Here's how the part is built. I have some questions about the finished solid (model axes, mm). Face numbers are marked on the shaded views. A direction names the side the tool comes from. Coordinates: 2 decimals unless noted, no trailing zeros. Write each loop counter-clockwise with the first axis right and the second up, starting at its lowest first coordinate (ties: lowest second). Pieces come first, ordered by that corner, then holes.
Autodesk Inventor part; units mm, degrees
ref_plane "YZ Plane" through (0, 0, 0) normal (1, 0, 0) x (0, 1, 0)
ref_plane "XZ Plane" through (0, 0, 0) normal (0, 1, 0) x (-1, 0, 0)
ref_plane "XY Plane" through (0, 0, 0) normal (0, 0, 1) x (1, 0, 0)
sketch "Sketch1" plane through (0, 0, 0) normal (0, 1, 0) x (-1, 0, 0)
  line L0 (110, -80) -> (-110, -80)
  line L1 (-110, -80) -> (-110, 80)
  line L2 (-110, 80) -> (110, 80)
  line L3 (110, 80) -> (110, -80)
  line L4 (320.2117, -53.5522) -> (168.036, -53.5522) construction
  line L5 (168.036, -53.5522) -> (168.036, 90.1689) construction
  line L6 (168.036, 90.1689) -> (320.2117, 90.1689) construction
  line L7 (320.2117, 90.1689) -> (320.2117, -53.5522) construction
  line L8 (124.3, -89.75) -> (-124.3, -89.75) construction
  line L9 (-124.3, -89.75) -> (-124.3, 89.75) construction
  line L10 (-124.3, 89.75) -> (124.3, 89.75) construction
  line L11 (124.3, 89.75) -> (124.3, -89.75) construction
  line L12 (124.3, -89.75) -> (-124.3, 89.75) construction
  line L13 (-124.3, -89.75) -> (124.3, 89.75) construction
  line L14 (-152.4, -107.95) -> (152.4, -107.95)
  line L15 (152.4, -107.95) -> (152.4, 107.95)
  line L16 (152.4, 107.95) -> (-152.4, 107.95)
  line L17 (-152.4, 107.95) -> (-152.4, -107.95)
  line L18 (-152.4, -107.95) -> (152.4, 107.95) construction
  line L19 (152.4, -107.95) -> (-152.4, 107.95) construction
  line L20 (177.8, 133.35) -> (177.8, -133.35)
  line L21 (177.8, -133.35) -> (-177.8, -133.35)
  line L22 (-177.8, -133.35) -> (-177.8, 133.35)
  line L23 (-177.8, 133.35) -> (177.8, 133.35)
  point P0 (0, 0)
  dimension "d11" = 220
  dimension "d12" = 160
  dimension "d15" = 248.6
  dimension "d16" = 179.5
  dimension "d18" = 304.8
  dimension "d19" = 215.9
  dimension "d22" = 25.4
extrude "Top" add sketch "Sketch1" along normal blind 25.4 contours L17 L16 L15 L14 | L20 L21 L22 L23
sketch "Sketch3" plane through (177.8, 0, 133.35) normal (1, 0, 0) x (0, 0, -1)
  line L0 (0, 0) -> (0, 25.4)
  line L1 (266.7, 0) -> (266.7, 25.4)
  line L2 (0, 0) -> (266.7, 0)
  line L3 (266.7, 0) -> (266.7, -266.7)
  line L4 (266.7, -266.7) -> (0, -266.7)
  line L5 (0, -266.7) -> (0, 0)
  point P0 (133.35, 0)
  dimension "d25" = 266.7
extrude "Right" add sketch "Sketch3" against normal blind 50.8
sketch "Sketch4" plane through (-177.8, 0, -133.35) normal (-1, 0, 0) x (0, 0, 1)
  line L0 (0, 0) -> (0, 25.4)
  line L1 (266.7, -266.7) -> (266.7, 0)
  line L2 (0, 0) -> (266.7, 0)
  line L3 (266.7, 0) -> (266.7, -266.7)
  line L4 (266.7, -266.7) -> (0, -266.7)
  line L5 (0, -266.7) -> (0, 0)
  point P0 (133.35, 0)
  dimension "d28" = 266.7
extrude "Left" add sketch "Sketch4" against normal blind 50.8
sketch "Sketch5" plane through (0, 0, 0) normal (1, 0, 0) x (0, 1, 0)
  line L0 (-266.7, -133.35) -> (25.4, -133.35)
  line L1 (-266.7, 133.35) -> (-266.7, -133.35)
  line L2 (0, -133.35) -> (-266.7, 133.35)
  line L3 (-266.7, 133.35) -> (-275.6803, 124.3697)
  line L4 (-275.6803, 124.3697) -> (-8.9803, -142.3303)
  line L5 (-8.9803, -142.3303) -> (0, -133.35)
  point P0 (0, 0)
  dimension "d31" = 12.7
extrude "Plexiglass Cut" cut sketch "Sketch5" along normal mid plane 304.8 contours L4 L1 L2 L0 | L0 L5 L4 | L4 L3 L1
sketch "Sketch6" plane through (-177.8, -266.7, -133.35) normal (0, -1, 0) x (1, 0, 0)
  line L0 (0, 0) -> (0, 266.7)
  line L1 (355.6, 0) -> (0, 0)
  line L2 (0, 266.7) -> (355.6, 266.7)
  line L3 (355.6, 266.7) -> (355.6, 0)
  line L4 (355.6, 0) -> (0, 0)
  line L5 (0, 0) -> (0, 266.7)
  point P0 (177.8, 133.35)
extrude "Bottom" add sketch "Sketch6" along normal blind 25.4
sketch "Sketch9" plane through (0, 25.4, 0) normal (0, 1, 0) x (1, 0, 0)
  line L0 (177.8, -133.35) -> (127, -133.35)
  line L1 (177.8, 133.35) -> (-177.8, 133.35)
  line L2 (177.8, -133.35) -> (-177.8, -133.35)
  line L3 (-177.8, -133.35) -> (-177.8, 133.35)
  line L4 (-177.8, 133.35) -> (177.8, 133.35)
  line L5 (177.8, 133.35) -> (177.8, -133.35)
  point P0 (0, 0)
extrude "Top Flattening" cut sketch "Sketch9" against normal blind 22.4
sketch "Sketch10" plane through (0, 3, 0) normal (0, 1, 0) x (1, 0, 0)
  line L0 (-177.8, -133.35) -> (-177.8, 133.35)
  line L1 (-155.4106, 133.35) -> (-177.8, 133.35)
  line L2 (-177.8, 133.35) -> (-177.8, -133.35)
  line L3 (-177.8, -133.35) -> (-155.4106, -133.35)
  line L4 (-155.4106, -133.35) -> (-155.4106, 133.35)
  line L5 (177.8, 133.35) -> (177.8, -133.35)
  line L6 (177.8, -133.35) -> (155.4106, -133.35)
  line L7 (155.4106, -133.35) -> (155.4106, 133.35)
  line L8 (155.4106, 133.35) -> (177.8, 133.35)
  line L9 (152.4, -115.3895) -> (152.4, 133.35)
  point P0 (0, 0)
  point P1 (-177.8, 0)
  dimension "d48" = 22.3894
  dimension "d49" = 22.3894
extrude "Outer Side Flattening" cut sketch "Sketch10" against normal through all
sketch "Sketch11" plane through (-177.8, -292.1, -133.35) normal (0, -1, 0) x (1, 0, 0)
  line L0 (22.3894, 0) -> (333.2106, 0)
  line L1 (333.2106, 0) -> (22.3894, 0)
  line L2 (22.3894, 0) -> (22.3894, 266.7)
  line L3 (22.3894, 266.7) -> (333.2106, 266.7)
  line L4 (333.2106, 266.7) -> (333.2106, 0)
  point P0 (177.8, 133.35)
extrude "Bottom Flattening" cut sketch "Sketch11" against normal blind 22.4
sketch "Sketch12" plane through (155.4106, 3, -133.35) normal (0, 0, -1) x (-1, 0, 0)
  line L0 (155.4106, -3) -> (155.4106, -269.7) construction
  line L1 (7.0106, -269.7) -> (7.0106, -3)
  line L2 (7.0106, -3) -> (303.8106, -3)
  line L3 (303.8106, -3) -> (303.8106, -269.7)
  line L4 (303.8106, -269.7) -> (7.0106, -269.7)
  line L5 (7.0106, -269.7) -> (303.8106, -3) construction
  line L6 (7.0106, -3) -> (303.8106, -269.7) construction
  point P0 (155.4106, -136.35)
  point P1 (155.4106, -3)
  dimension "d54" = 296.8
extrude "Inner Flattening" cut sketch "Sketch12" against normal through all
sketch "Sketch13" plane through (-155.4106, 3, 133.35) normal (0, 0, 1) x (1, 0, 0)
  line L0 (310.8211, -272.7) -> (310.8211, 0)
  line L1 (0, -272.7) -> (0, 0)
  line L2 (310.8211, -136.35) -> (0, -136.35)
  line L3 (0, -136.35) -> (0, 0)
  line L4 (0, 0) -> (310.8211, 0)
  line L5 (310.8211, 0) -> (310.8211, -136.35)
  point P0 (155.4106, -3)
  point P1 (310.8211, 0)
  point P2 (0, -136.35)
extrude "Top Cut" cut sketch "Sketch13" against normal through all
sketch "Sketch14" plane through (-155.4106, -133.35, 133.35) normal (0, 1, 0) x (1, 0, 0)
  line L0 (310.8212, 0) -> (303.8106, 0)
  line L1 (155.4106, 133.35) -> (310.8212, 133.35)
  line L2 (310.8212, 133.35) -> (310.8212, 0)
  line L3 (310.8212, 0) -> (155.4106, 0)
  line L4 (155.4106, 0) -> (155.4106, 133.35)
  line L5 (310.8211, 266.7) -> (0, 266.7)
  line L6 (310.8212, 0) -> (0, 0)
  line L7 (0, 0) -> (0, 266.7)
  line L8 (0, 266.7) -> (310.8212, 266.7)
  line L9 (310.8212, 266.7) -> (310.8212, 0)
extrude "Quarter Cut" cut sketch "Sketch14" against normal through all contours L1 L4 L6 L7 L5 L9
properties part number "Apple iPad 2022 Hologram"
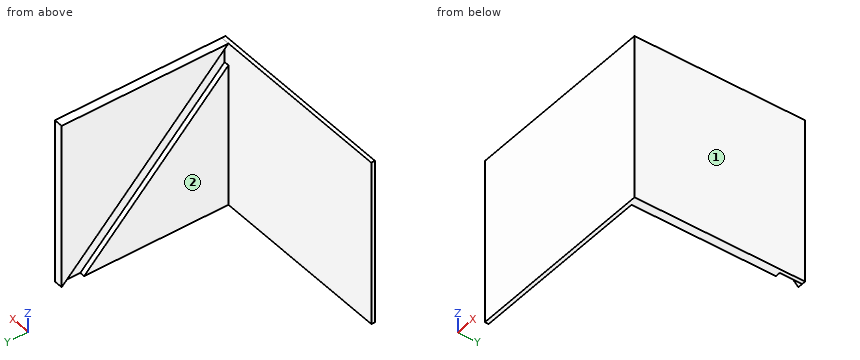
1) On a 3-axis mill with a long thin cutter (end or side, diameter ignored), from which of +Z, -Z, +X, -X, +Y, -Y can I reach the whole of each face in a straight line? I mean the marked faces 1 and 2. Say none if no direction works.
Values follow:
face 1: +Z, -Z, +X, +Y, -Y
face 2: +Z, -Z, -X, +Y
2) I need wall thicknesses on probe 1 along X at (y, z) = (-207, 33); probe 2 along Y at (x, z) = (108, 86.5); probe 3 along X at (y, z) = (-192.5, 54). Which ranges of each line are inside material? Lowest first, please.
Values follow:
probe 1: x = 148.4 to 155.41
probe 2: y = -269.7 to -266.7
probe 3: x = 152.4 to 155.41
3) Imagine slicing it at D-D on y = -233.5. Please give me the cut outline in (x, z).
Values follow:
outline: (148.4, 0) - (155.41, 0) - (155.41, 133.35) - (148.4, 133.35) - (148.4, 100.15) - (152.4, 100.15) - (152.4, 82.19) - (148.4, 82.19) - close
4) Imagine slicing it at B-B on x = 18.5. Please give me the cut outline in (y, z), then the cut area to 3 significant figures.
Values follow:
outline: (-269.7, 0) - (-266.7, 0) - (-266.7, 133.35) - (-269.7, 133.35) - close
area: 400 mm2
5) Will these pins go through, and if not, where does the flat tip stop? pin 1 (12 mm diameter, centred on y = -235, z = 72.5, fed in from -X); pin 2 (8 mm diameter, centred on x = 121.5, z = 67, fed in from +Y).
Values follow:
pin 1: stops at x = 148.4
pin 2: stops at y = -266.7
6) Imagine slicing it at A-A on y = -142.5. Please give me the cut outline in (x, z).
Values follow:
outline: (148.4, 9.15) - (152.4, 9.15) - (152.4, 0) - (155.41, 0) - (155.41, 133.35) - (148.4, 133.35) - close
7) Imagine slicing it at C-C on z = 43.5. Please give me the cut outline in (x, y), then the cut area to 3 significant figures.
Values follow:
outline: (0, -269.7) - (155.41, -269.7) - (155.41, -133.35) - (148.4, -133.35) - (148.4, -176.85) - (152.4, -176.85) - (152.4, -194.81) - (148.4, -194.81) - (148.4, -266.7) - (0, -266.7) - close
area: 1,330 mm2
